Model file for the job. Use its own axes, mm. A direction names the side the tool comes from. Round coordinates to 2 decimals unless told otherwise and drop trailing zeros. Loops run counter-clockwise (first coordinate to the right, second up) from the corner with the lowest first, then second, coordinate; pieces in that order, holes last. Notation, with made-up numbers: (41.25, 58) -> (90.25, 58) arc R26 ccw to (90.25, 95) -> close; hole circle Ø2 at (69.5, 82). An arc over 180 degrees is marked (long way). Use a Markdown table: item, result.
from build123d import *

# Parameters (mm, degrees)
SKETCH1_W               = 19
SKETCH1_H               = 44
BOSS_EXTRUDE1_DEPTH     = 14
CUT_EXTRUDE1_DEPTH      = 48.140746706
CUT_EXTRUDE1_DEPTH_BACK = 48.140746706
SKETCH2_R               = 1.5
CUT_EXTRUDE2_START      = -9.5
SKETCH3_R               = 1.5
CUT_EXTRUDE2_DEPTH      = 20
BOSS_EXTRUDE2_START     = 14
SKETCH4_W               = 19
SKETCH4_H               = 4
BOSS_EXTRUDE2_DEPTH     = 3
CUT_EXTRUDE3_START      = 17
SKETCH5_R               = 1.15
CUT_EXTRUDE3_DEPTH      = 7.5
SKETCH6_R               = 3
CUT_EXTRUDE4_DEPTH      = 9.5
CUT_EXTRUDE5_DEPTH      = 49.117044817
CUT_EXTRUDE5_DEPTH_BACK = 49.117044817
SKETCH8_R               = 1.5
CUT_EXTRUDE6_DEPTH      = 36
SKETCH9_R               = 5
CUT_EXTRUDE7_DEPTH      = 2


with BuildPart() as part:
    # Sketch1 → Boss-Extrude1 (new body)
    with BuildSketch(Plane.XY):
        with Locations((0, 22)):
            Rectangle(SKETCH1_W, SKETCH1_H)
    extrude(amount=BOSS_EXTRUDE1_DEPTH)

    # Sketch2 → Cut-Extrude1 (cut, two sides: drawn at the far end of the back side and taken through both)
    with BuildSketch(Plane.XY.offset(-CUT_EXTRUDE1_DEPTH_BACK)):
        with Locations((0, 2)):
            Circle(SKETCH2_R)
        with Locations((0, 42)):
            Circle(SKETCH2_R)
    extrude(amount=CUT_EXTRUDE1_DEPTH + CUT_EXTRUDE1_DEPTH_BACK, mode=Mode.SUBTRACT)

    # Sketch3 → Cut-Extrude2 (cut)
    with BuildSketch(Plane(origin=(0, 0, 0), x_dir=(0, 0, -1), z_dir=(1, 0, 0)).offset(CUT_EXTRUDE2_START)):
        with Locations(Location((-7, 7.5, 0), (0, 0, 180))):
            Circle(SKETCH3_R)
        with Locations(Location((-7, 38.5, 0), (0, 0, 180))):
            Circle(SKETCH3_R)
        with Locations(Location((-2.5, 3.5, 0), (0, 0, 180))):
            Circle(SKETCH3_R)
        with Locations(Location((-2.5, 34.5, 0), (0, 0, 180))):
            Circle(SKETCH3_R)
    extrude(amount=CUT_EXTRUDE2_DEPTH, mode=Mode.SUBTRACT)

    # Sketch4 → Boss-Extrude2 (add)
    with BuildSketch(Plane.XY.offset(BOSS_EXTRUDE2_START)):
        with Locations((0, 29)):
            Rectangle(SKETCH4_W, SKETCH4_H)
    extrude(amount=BOSS_EXTRUDE2_DEPTH)

    # Sketch5 → Cut-Extrude3 (cut)
    with BuildSketch(Plane.XY.offset(CUT_EXTRUDE3_START)):
        with Locations((-0.5, 29)):
            Circle(SKETCH5_R)
    extrude(amount=-CUT_EXTRUDE3_DEPTH, mode=Mode.SUBTRACT)

    # Sketch6 → Cut-Extrude4 (cut)
    with BuildSketch(Plane.XY):
        with Locations((-0.5, 29)):
            Circle(SKETCH6_R)
    extrude(amount=CUT_EXTRUDE4_DEPTH, mode=Mode.SUBTRACT)

    # Sketch7 → Cut-Extrude5 (cut, two sides: drawn at the far end of the back side and taken through both)
    with BuildSketch(Plane.XY.offset(-CUT_EXTRUDE5_DEPTH_BACK)):
        Polygon((97.397368474, 34), (9.5, 34), (7.5, 34), (7.5, 12), (9.5, 12), (97.397368474, 12), (273.192105422, 12), (273.192105422, 34), align=None)
    extrude(amount=CUT_EXTRUDE5_DEPTH + CUT_EXTRUDE5_DEPTH_BACK, mode=Mode.SUBTRACT)

    # Sketch8 → Cut-Extrude6 (cut)
    with BuildSketch(Plane(origin=(0, 0, 0), x_dir=(-1, 0, 0), z_dir=(0, 0, -1))):
        with Locations((2.5, 10)):
            Circle(SKETCH8_R)
    extrude(amount=-CUT_EXTRUDE6_DEPTH, mode=Mode.SUBTRACT)

    # Sketch9 → Cut-Extrude7 (cut)
    with BuildSketch(Plane.XY.offset(14)):
        with Locations((-2.5, 10)):
            Circle(SKETCH9_R)
    extrude(amount=-CUT_EXTRUDE7_DEPTH, mode=Mode.SUBTRACT)


solid = part.part
Q1. Band-saw the part on D-D, the plane z = 11.25. Give the cut face in (x, y).
Results list:
| item | result |
|---|---|
| outline | (-9.5, 0) -> (9.5, 0) -> (9.5, 12) -> (7.5, 12) -> (7.5, 34) -> (9.5, 34) -> (9.5, 44) -> (-9.5, 44) -> close; hole circle Ø3 at (-2.5, 10); hole circle Ø2.3 at (-0.5, 29); hole circle Ø3 at (0, 2); hole circle Ø3 at (0, 42) |
Q2. Band-saw the part on B-B, the plane y = 29. Give the cut face in (x, z).
Results list:
| item | result |
|---|---|
| outline | (-9.5, 0) -> (-3.5, 0) -> (-3.5, 9.5) -> (-1.65, 9.5) -> (-1.65, 17) -> (-9.5, 17) -> close; (0.65, 9.5) -> (2.5, 9.5) -> (2.5, 0) -> (7.5, 0) -> (7.5, 17) -> (0.65, 17) -> close |
Q3. Band-saw the part on A-A, the plane z = 6. Give the cut face in (x, y), plus the area to 3 significant figures.
Results list:
| item | result |
|---|---|
| outline | (-9.5, 0) -> (9.5, 0) -> (9.5, 6.38) -> (-9.5, 6.38) -> close; (-9.5, 8.62) -> (-3.08, 8.62) arc R1.5 cw (long way) to (-1.92, 8.62) -> (9.5, 8.62) -> (9.5, 12) -> (7.5, 12) -> (7.5, 34) -> (9.5, 34) -> (9.5, 37.38) -> (-9.5, 37.38) -> close; (-9.5, 39.62) -> (9.5, 39.62) -> (9.5, 44) -> (-9.5, 44) -> close; hole circle Ø6 at (-0.5, 29); hole circle Ø3 at (0, 2); hole circle Ø3 at (0, 42) |
| area | 658 mm² |
Q4. Band-saw the part on C-C, the plane x = 0. Give the number of separate pieces and of enclosed holes in the cut face, plus the area to 3 significant figures.
Results list:
| item | result |
|---|---|
| separate pieces | 4 |
| enclosed holes | 3 |
| area | 430 mm² |
Q5. Drill centre lines: L1, parallel to Z at x = -4.25, y = 3.5; L2, parallel to Z at x = 7.25, y = 34; L3, parallel to Y at x = 7.75, z = 5.25. Where is each one in solid material? Low to high. Write a range as from..to.
Results list:
| item | result |
|---|---|
| L1 | z = 0..1, 4..14 |
| L2 | z = 0..1.09, 3.91..14 |
| L3 | y = 0..12, 34..44 |
Q6. Flat gauge pins, fed straight in: pin 1 (8 mm diameter, centred on x = -7.5, z = 12, fed in from -Y); pin 2 (11 mm diameter, centred on x = -1.5, y = 8.5, fed in from +Z); pin 3 (1.8 mm diameter, centred on y = 7.5, z = 7, fed in from +X); pin 4 (0.9 mm diameter, centred on x = 0.5, z = 16, fed in from -Y). Where does each tip first touch, or does it go through?
Results list:
| item | result |
|---|---|
| pin 1 | stops at y = 0 |
| pin 2 | stops at z = 14 |
| pin 3 | passes through |
| pin 4 | stops at y = 27 |
Q7. Pull direction Y, two halves, no side cores. Call faces 4 (the face through (0, 6, 7)), 5 (the face through (0, 44, 7)), 6 (the face through (9.5, 40, 8)): released by +Y, released by -Y, zero draft, split by the parting line, or undercut.
Results list:
| item | result |
|---|---|
| face 4 | undercut |
| face 5 | released by +Y |
| face 6 | zero draft |
Q8. Tool access for faces 1 (the face through (-1.15, 26.07, 4.68)), 2 (the face through (-4, 9, 12)), 3 (the face through (8, 12, 7)): list every direction of +Z, -Z, +X, -X, +Y, -Y with a clear straight run to the whole face (end or side of a thin tool).
Results list:
| item | result |
|---|---|
| face 1 | -Z |
| face 2 | +Z |
| face 3 | +Z, -Z, +X |
